```python
from build123d import *

# Parameters (mm, degrees)
BOSS_EXTRUDE1_DEPTH = 6.35
SKETCH2_R           = 3.4925
SKETCH2_R_2         = 3.556
CUT_EXTRUDE1_DEPTH  = 6.35
FILLET1_R           = 2.54


with BuildPart() as part:
    # Sketch1 → Boss-Extrude1 (new body)
    with BuildSketch(Plane.XY):
        Polygon((38.1, -38.1), (76.2, 0), (76.2, 38.1), (0, 38.1), (0, 0), (0, -38.1), align=None)
    extrude(amount=BOSS_EXTRUDE1_DEPTH)

    # Sketch2 → Cut-Extrude1 (cut)
    with BuildSketch(Plane.XY.offset(6.35)):
        with Locations((19.05, 19.05)):
            Circle(SKETCH2_R)
        with Locations((57.15, 19.05)):
            Circle(SKETCH2_R)
        with Locations((19.05, -19.05)):
            Circle(SKETCH2_R_2)
    extrude(amount=-CUT_EXTRUDE1_DEPTH, mode=Mode.SUBTRACT)

    # Fillet1
    fillet1_edges = [part.edges().sort_by_distance(p)[0] for p in [
        (57.15, -19.05, 6.35),
        (76.2, 19.05, 6.35),
        (38.1, 38.1, 6.35),
        (0, 0, 6.35),
        (19.05, -38.1, 6.35),
    ]]
    fillet(fillet1_edges, radius=FILLET1_R)


solid = part.part
```
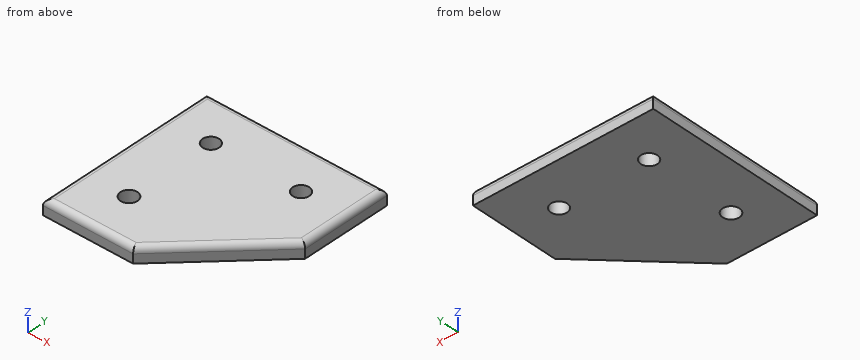
Source: CAD feature listing. Evaluate the final solid. Frame: model axes, mm. Coordinates: 2 decimals unless noted, no trailing zeros. Write each loop counter-clockwise with the first axis right and the second up, starting at its lowest first coordinate (ties: lowest second). Pieces come first, ordered by that corner, then holes. Notation, with made-up numbers: (82.25, -4) -> (100.25, -4) arc R22 cw to (100.25, 30) -> close; hole circle Ø4 at (35, -4.75). An arc over 180 degrees is marked (long way). Return JSON: item names as keys, results as strings. Group by question number.
1) Section query B-B, the plane x = 19.05. Return loops of the section in (y, z), plus the area to 3 significant figures.
2) Ray query, line 1 along Y through (x, z) = (19.05, 4); line 2 along X through (y, z) = (18, 4); line 3 along Y through (x, z) = (19.05, 4.5). Return the intervals inside material, ascending.
3) Contact query for a flat-ended pin moving along its axis: P1, Ø2, axis at x = 24, z = 5, coming from the +Y side. Output: stop coordinate, or through.
4) Section query A-A, the plane y = 19.05. Return loops of the section in (x, z), plus the area to 3 significant figures.
5) Section query C-C, the plane z = 1.75. State how many separate pieces and enclosed holes the cut face has, plus the area to 3 significant figures.
From the geometry:
{
 "1": {"outline": "(-38.1, 0) -> (-22.61, 0) -> (-22.61, 6.35) -> (-35.56, 6.35) arc R2.54 ccw to (-38.1, 3.81) -> close; (-15.49, 0) -> (15.56, 0) -> (15.56, 6.35) -> (-15.49, 6.35) -> close; (22.54, 0) -> (38.1, 0) -> (38.1, 3.81) arc R2.54 ccw to (35.56, 6.35) -> (22.54, 6.35) -> close", "area": "392 mm²"},
 "2": {"line 1": "-38.09 to -22.61, -15.49 to 15.56, 22.54 to 38.09", "line 2": "0.01 to 15.72, 22.38 to 53.82, 60.48 to 76.19", "line 3": "-38 to -22.61, -15.49 to 15.56, 22.54 to 38"},
 "3": {"P1": "y = 38.09"},
 "4": {"outline": "(0, 0) -> (15.56, 0) -> (15.56, 6.35) -> (2.54, 6.35) arc R2.54 ccw to (0, 3.81) -> close; (22.54, 0) -> (53.66, 0) -> (53.66, 6.35) -> (22.54, 6.35) -> close; (60.64, 0) -> (76.2, 0) -> (76.2, 3.81) arc R2.54 ccw to (73.66, 6.35) -> (60.64, 6.35) -> close", "area": "392 mm²"},
 "5": {"separate pieces": "1", "enclosed holes": "3", "area": "4,960 mm²"}
}
